Autodesk Fusion 360 part; units mm, degrees
sketch "Sketch1" plane through (0, 0, 0) normal (0, 1, 0) x (1, 0, 0)
  line L0 (67, -50) -> (-47, -50)
  line L1 (-47, -50) -> (-47, 90)
  line L2 (-47, 90) -> (-35, 90)
  line L3 (-35, 90) -> (-35, 52)
  line L4 (-35, 52) -> (67, 52)
  line L5 (67, 52) -> (67, -50)
  line L6 (65.2, -48.2) -> (-45.2, -48.2)
  line L7 (-45.2, -48.2) -> (-45.2, 88.2)
  line L8 (-45.2, 88.2) -> (-36.8, 88.2)
  line L9 (-36.8, 88.2) -> (-36.8, 50.2)
  line L10 (-36.8, 50.2) -> (65.2, 50.2)
  line L11 (65.2, 50.2) -> (65.2, -48.2)
  dimension "d1" = 102
  dimension "d3" = 140
  dimension "d4" = 12
  dimension "d5" = 102
  dimension "d6" = 1.8
extrude "Extrude1" add sketch "Sketch1" along normal blind 2.5 contours L0 L1 L2 L3 L4 L5 | L6 L7 L8 L9 L10 L11
sketch "Sketch2" plane through (0, 2.5, 0) normal (0, 1, 0) x (-1, 0, 0)
  line L0 (-67, -52) -> (35, -52)
  line L1 (35, -52) -> (35, -90)
  line L2 (35, -90) -> (47, -90)
  line L3 (47, -90) -> (47, 50)
  line L4 (47, 50) -> (-67, 50)
  line L5 (-67, 50) -> (-67, -52)
  line L6 (37.8, -87.2) -> (44.2, -87.2)
  line L7 (44.2, -87.2) -> (44.2, 47.2)
  line L8 (44.2, 47.2) -> (-64.2, 47.2)
  line L9 (-64.2, 47.2) -> (-64.2, -49.2)
  line L10 (-64.2, -49.2) -> (37.8, -49.2)
  line L11 (37.8, -49.2) -> (37.8, -87.2)
  dimension "d9" = -2.8
extrude "Extrude2" add sketch "Sketch2" along normal blind 2.5 contours L6 L7 L8 L9 L10 L11
sketch "Sketch3" plane through (0, 5, 0) normal (0, 1, 0) x (-1, 0, 0)
  line L0 (37.8, -49.2) -> (37.8, -87.2)
  line L1 (37.8, -87.2) -> (44.2, -87.2)
  line L2 (44.2, -87.2) -> (44.2, 47.2)
  line L3 (44.2, 47.2) -> (-64.2, 47.2)
  line L4 (-64.2, 47.2) -> (-64.2, -49.2)
  line L5 (-64.2, -49.2) -> (37.8, -49.2)
  line L6 (16.8, -40.8) -> (16.8, 42.2)
  line L7 (16.8, 42.2) -> (-49.2, 42.2)
  line L8 (-49.2, 42.2) -> (-49.2, -40.8)
  line L9 (-49.2, -40.8) -> (-46.2, -40.8)
  line L10 (-46.2, -40.8) -> (-46.2, 39.2)
  line L11 (-46.2, 39.2) -> (13.8, 39.2)
  line L12 (13.8, 39.2) -> (13.8, -40.8)
  line L13 (13.8, -40.8) -> (16.8, -40.8)
  dimension "d12" = 60
  dimension "d13" = 80
  dimension "d14" = 3
  dimension "d15" = 3
  dimension "d16" = 3
  dimension "d17" = 5
  dimension "d18" = 15
extrude "Extrude3" add sketch "Sketch3" along normal blind 5 contours L6 L7 L8 L9 L10 L11 L12 L13
equation "d15 = d14"
equation "d16 = d14"
Verification items for the finished model (mm, model axes). A direction names the side the tool comes from. Give positions to 0.01 mm unless a question says otherwise; leave off trailing zeros. Write each loop counter-clockwise with the first axis right and the second up, starting at its lowest first coordinate (ties: lowest second). Pieces come first, ordered by that corner, then holes.
(1) Cross-section at C-C (x = 36). Enter the section's corners in (y, z).
(2) Mould release check, pull along X, two halves, no side actions. Record for faces 1 (the face through (-13.8, 7, 0)), 2 (the face through (-16.8, 7, 0)), 3 (the face through (16, 7, 42.2)): +X half, -X half, draft (parallel to the pull), parting line (faces both ways), or undercut.
(3) Material ranges on line 1 (X direction, y = 7, z = -30.5); line 2 (Z direction, x = 1.5, y = 0.75); line 3 (Y direction, x = 9, z = 7), recorded low to high.
(4) Access from +Z, -Z, +X, -X, +Y, -Y to the whole of each face (thin tool, end or side, straight path). Record for faces 4 (the face through (49.2, 7, 1)), 5 (the face through (9, 0, -5)), 6 (the face through (17, 7, 39.2)), 7 (the face through (16, 10, 41)), 8 (the face through (-15, 7, -40.8)).
(5) Gauge pin test, flat ends, axial feed: pin 1 (2.5 mm diameter, centred on y = 6.5, z = -10, fed in from +X); pin 2 (0.8 mm diameter, centred on y = 1, z = -69.5, fed in from +X); pin 3 (4 mm diameter, centred on x = 28.5, y = 6, fed in from -Z); pin 4 (5 mm diameter, centred on x = -34, y = 1, fed in from -Z). Record the tip position at first contact, or that the pin passes through.
(6) Cross-section at A-A (z = -17). Enter the section's corners in (x, y), plus the area to 3 significant figures.
(7) Cross-section at B-B (y = 7). Enter the section's corners in (x, z), plus the area to 3 significant figures.
(8) Cross-section at D-D (z = -47.5). Enter the section's corners in (x, y), plus the area to 3 significant figures.
Worked out:
1. outline: (0, -52) - (2.5, -52) - (2.5, -49.2) - (5, -49.2) - (5, 39.2) - (10, 39.2) - (10, 42.2) - (5, 42.2) - (5, 47.2) - (2.5, 47.2) - (2.5, 50) - (0, 50) - close
2. face 1: undercut
2. face 2: -X half
2. face 3: draft
3. line 1: x = -16.8 to -13.8, 46.2 to 49.2
3. line 2: z = -52 to 50
3. line 3: y = 0 to 5
4. face 4: +Z, -Z, +X, +Y
4. face 5: +Z, -Z, +X, -X, -Y
4. face 6: -Z, +Y
4. face 7: +Z, -Z, +X, -X, +Y
4. face 8: -Z, +X, -X, +Y
5. pin 1: stops at x = 49.2
5. pin 2: stops at x = -35
5. pin 3: stops at z = -49.2
5. pin 4: stops at z = -90
6. outline: (-47, 0) - (67, 0) - (67, 2.5) - (64.2, 2.5) - (64.2, 5) - (49.2, 5) - (49.2, 10) - (46.2, 10) - (46.2, 5) - (-13.8, 5) - (-13.8, 10) - (-16.8, 10) - (-16.8, 5) - (-44.2, 5) - (-44.2, 2.5) - (-47, 2.5) - close
6. area: 586 mm2
7. outline: (-16.8, -40.8) - (-13.8, -40.8) - (-13.8, 39.2) - (46.2, 39.2) - (46.2, -40.8) - (49.2, -40.8) - (49.2, 42.2) - (-16.8, 42.2) - close
7. area: 678 mm2
8. outline: (-47, 0) - (67, 0) - (67, 2.5) - (64.2, 2.5) - (64.2, 5) - (-44.2, 5) - (-44.2, 2.5) - (-47, 2.5) - close
8. area: 556 mm2
